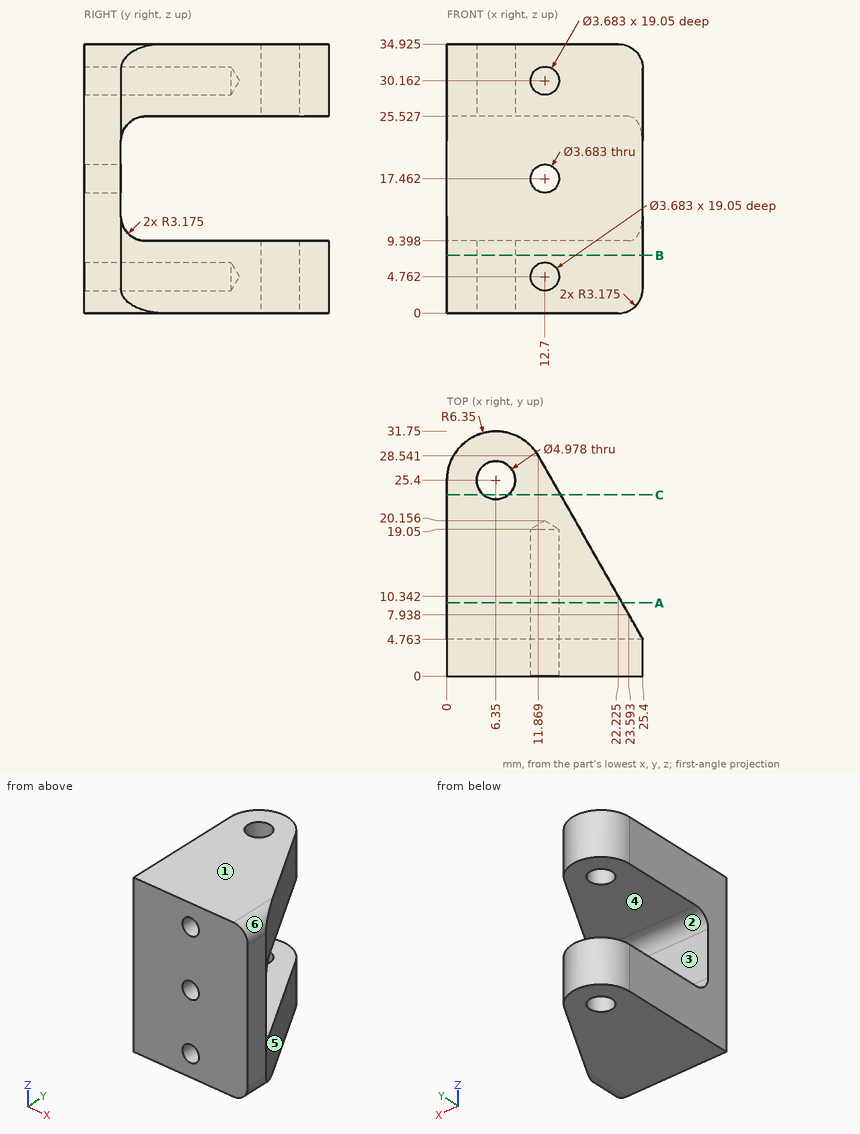
For this review, use the dimensioned drawing (mm, ordinates from the lowest corner) and the shaded views. A direction names the side the tool comes from. Coordinates: 2 decimals unless noted, no trailing zeros. Write each loop counter-clockwise with the first axis right and the second up, starting at its lowest first coordinate (ties: lowest second). Pieces come first, ordered by that corner, then holes. Notation, with made-up numbers: (15.25, 67.5) -> (57.25, 67.5) arc R20 ccw to (57.25, 73.5) -> close; hole circle Ø3 at (11.25, 43). An arc over 180 degrees is marked (long way). Put each result on its own line as item: value.
Q1. The part is to be moulded in two halves that separate along Z. For the marked faces 3, 4, 5 and 6, say which applies: +Z half, -Z half, draft (parallel to the pull), parting line (faces both ways), or undercut.
From the geometry:
face 3: undercut
face 4: undercut
face 5: draft
face 6: +Z half
Q2. Clearance check with flat-ended pins moving along their axes: pin 1 Ø5.5 at (x, y) = (6.35, 25.4) entering from -Z; pin 2 Ø3.5 at (x, z) = (12.7, 17.46) entering from +Y; pin 3 Ø10 at (x, z) = (12.5, 28) entering from +Y (1 decimal); pin 4 Ø3.5 at (x, z) = (12.7, 30.16) entering from -Y. State where each tip first meets the part, or that it passes through.
From the geometry:
pin 1: stops at z = 0
pin 2: passes through
pin 3: stops at y = 31.6
pin 4: stops at y = 19.1
Q3. Wall thickness on L1, parallel to Z at x = 12.7, y = 8.75 (1 decimal); L2, parallel to Z at x = 12.7, y = 3.1 (1 decimal); L3, parallel to Z at x = 9.5, y = 21 (1 decimal): over which ranges is each line inside the solid? List them lowest first.
From the geometry:
L1: z = 0 to 2.9, 6.6 to 9.4, 25.5 to 28.3, 32 to 34.9
L2: z = 0 to 2.9, 6.6 to 15.6, 19.3 to 28.3, 32 to 34.9
L3: z = 0 to 9.4, 25.5 to 34.9
Q4. Take a section at A-A, the plane y = 9.5. Count the separate pieces of the cut face and the enclosed holes in it.
From the geometry:
separate pieces: 2
enclosed holes: 2
Q5. Tool access review of the marked faces 1 and 2: name each direction out of +Z, -Z, +X, -X, +Y, -Y from which nothing blocks a thin tool from reaching the whole face with its end or side.
From the geometry:
face 1: +Z, +X, -X, +Y, -Y
face 2: +X, -X, +Y
Q6. Take a section at C-C, the plane y = 23.5. State the section outline as (x, z) points (1 decimal).
From the geometry:
outline: (0, 0) -> (4.7, 0) -> (4.7, 9.4) -> (0, 9.4) -> close; (0, 25.5) -> (4.7, 25.5) -> (4.7, 34.9) -> (0, 34.9) -> close; (8, 0) -> (14.7, 0) -> (14.7, 9.4) -> (8, 9.4) -> close; (8, 25.5) -> (14.7, 25.5) -> (14.7, 34.9) -> (8, 34.9) -> close
Q7. Take a section at B-B, the plane z = 7.5. State the section outline as (x, y) points.
From the geometry:
outline: (0, 0) -> (25.4, 0) -> (25.4, 4.76) -> (11.87, 28.54) arc R6.35 ccw to (0, 25.4) -> close; hole circle Ø4.98 at (6.35, 25.4)
